Can you work these out from the model? Positions are in its coordinate system, mm. Face numbers are marked on the shaded views. A direction names the side the tool comes from. Give positions to 0.01 mm unless a question says otherwise; leave off trailing zeros. Write each loop counter-clockwise with the first axis right and the second up, starting at its lowest first coordinate (ties: lowest second). Pieces come first, ordered by that corner, then holes. Notation, with made-up numbers: (-16, 8) - (34, 8) arc R26 ccw to (34, 25) - close; hole circle Ø4 at (4, -9.5). An arc over 180 degrees is marked (long way). Return JSON: item names as keys, results as strings. Group by question number.
from build123d import *

# Parameters (mm, degrees)
BOSS_EXTRUDE1_DEPTH = 5
BOSS_EXTRUDE2_DEPTH = 30


with BuildPart() as part:
    # Sketch1 → Boss-Extrude1 (new body)
    with BuildSketch(Plane(origin=(0, 0, 0), x_dir=(1, 0, 0), z_dir=(0, 1, 0))):
        Polygon((13, 50), (5, 50), (5, 5), (50, 5), (50, 13), (13, 13), align=None)
    extrude(amount=BOSS_EXTRUDE1_DEPTH)

    # Sketch1<3> → Boss-Extrude2 (add)
    with BuildSketch(Plane(origin=(0, 0, 0), x_dir=(1, 0, 0), z_dir=(0, 1, 0))):
        Polygon((0, 50), (0, 0), (50, 0), (50, 5), (5, 5), (5, 50), align=None)
        Polygon((18, 50), (13, 50), (13, 13), (50, 13), (50, 18), (18, 18), align=None)
    extrude(amount=BOSS_EXTRUDE2_DEPTH)


solid = part.part
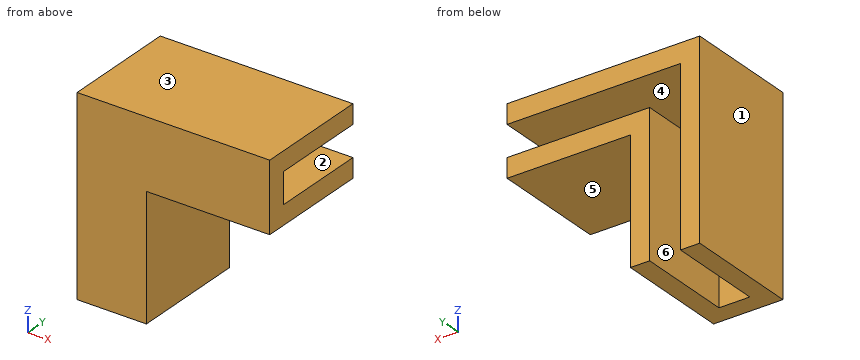
1) Will these pins go through, and if not, where does the flat tip stop? pin 1 Ø9 at (x, y) = (33, 11) entering from -Z; pin 2 Ø15 at (y, z) = (22.5, -33.5) entering from +X; pin 3 Ø2 at (y, z) = (15, -10.5) entering from +X.
2) Imagine slicing it at A-A, the plane y = 7.25. Write out the boundary of the cut face in (x, z), and give its area (3 significant figures).
3) I need wall thicknesses on line 1 along X through (y, z) = (22.25, -37); line 2 along X through (y, z) = (13.75, -16.5); line 3 along Z through (x, y) = (23.5, 13.25). Which ranges of each line are inside material? Lowest first, please.
4) Imagine slicing it at B-B, the plane x = 29. Write out the boundary of the cut face in (y, z), and give its area (3 significant figures).
5) Imagine slicing it at C-C, the plane z = -41. Write out the boundary of the cut face in (x, y).
6) We'd pull the mould along Z, two halves only. Please class the marked faces 1, 2 and 3: pulls with the +Z half, pulls with the -Z half, needs draft (parallel to the pull), parting line crosses it, or undercut.
7) Imagine slicing it at D-D, the plane y = 3. Write out the boundary of the cut face in (x, z), and give its area (3 significant figures).
8) On a 3-axis mill with a long thin cutter (end or side, diameter ignored), from which of +Z, -Z, +X, -X, +Y, -Y can I reach the whole of each face in a straight line? I mean the marked faces 4, 5 and 6. Say none if no direction works.
Resolved:
{
 "1": {"pin 1": "z = -18", "pin 2": "x = 18", "pin 3": "x = 5"},
 "2": {"outline": "(0, -50) - (5, -50) - (5, -5) - (50, -5) - (50, 0) - (0, 0) - close; (13, -50) - (18, -50) - (18, -18) - (50, -18) - (50, -13) - (13, -13) - close", "area": "820 mm^2"},
 "3": {"line 1": "0 to 5, 13 to 18", "line 2": "0 to 5, 13 to 50", "line 3": "-18 to -13, -5 to 0"},
 "4": {"outline": "(0, -18) - (30, -18) - (30, -13) - (5, -13) - (5, -5) - (30, -5) - (30, 0) - (0, 0) - close", "area": "340 mm^2"},
 "5": {"outline": "(0, 0) - (18, 0) - (18, 30) - (13, 30) - (13, 5) - (5, 5) - (5, 30) - (0, 30) - close"},
 "6": {"face 1": "needs draft", "face 2": "undercut", "face 3": "pulls with the +Z half"},
 "7": {"outline": "(0, -50) - (18, -50) - (18, -18) - (50, -18) - (50, 0) - (0, 0) - close", "area": "1,480 mm^2"},
 "8": {"face 4": "+X, +Y", "face 5": "-Z, +X, +Y, -Y", "face 6": "-Z, +Y"}
}
